CAD build for the part. Positions are in the model's coordinates, mm. A direction names the side the tool comes from. Coordinates: 2 decimals unless noted, no trailing zeros. Order: outer loops, then holes, each group sorted by start corner. A loop starts at its lowest first (then second) coordinate and runs counter-clockwise, first axis right, second up. Notation, with made-up numbers: M 12.25,15 L 35.25,15 A7 ccw 35.25,27 Z; hole C 45.5,25.5 d3. An arc over 180 degrees is marked long. One line per item, written item: value.
Autodesk Inventor part; units mm, degrees
ref_plane "YZ Plane" through (0, 0, 0) normal (1, 0, 0) x (0, 1, 0)
ref_plane "XZ Plane" through (0, 0, 0) normal (0, 1, 0) x (-1, 0, 0)
ref_plane "XY Plane" through (0, 0, 0) normal (0, 0, 1) x (1, 0, 0)
sketch "Sketch1" plane through (0, 0, 0) normal (0, 0, 1) x (1, 0, 0)
  point P0 (0, 0)
sketch "Sketch2" plane through (0, 0, 0) normal (0, 0, 1) x (1, 0, 0)
  line L0 (76.1957, 14.1695) -> (-73.6643, 14.1695) construction
  line L1 (-73.6643, -54.4105) -> (76.1957, -54.4105) construction
  line L2 (34.477, 19.1695) -> (24.477, 19.1695)
  line L3 (24.477, -59.4105) -> (34.477, -59.4105)
  line L4 (34.477, -59.4105) -> (34.477, 19.1695)
  line L5 (24.477, -15.1205) -> (-78.6643, -15.1205)
  line L6 (-78.6643, -15.1205) -> (-78.6643, -25.1205)
  line L7 (-78.6643, -25.1205) -> (24.477, -25.1205)
  line L8 (-73.6643, 14.1695) -> (-73.6643, -54.4105) construction
  line L9 (76.1957, -54.4105) -> (76.1957, 14.1695) construction
  line L10 (76.1957, -20.1205) -> (-73.6643, -20.1205) construction
  line L11 (24.477, 19.1695) -> (24.477, -15.1205)
  line L12 (24.477, -25.1205) -> (24.477, -59.4105)
  line L13 (44.477, -30.2805) -> (44.477, -9.9605) construction
  line L14 (57.177, -30.2805) -> (44.477, -30.2805) construction
  line L15 (57.177, -9.9605) -> (57.177, -30.2805) construction
  line L16 (44.477, -9.9605) -> (57.177, -9.9605) construction
  point P0 (0, 0)
  point P1 (-78.6643, -20.1205)
  dimension "d0" = 5
  dimension "d1" = 5
  dimension "d2" = 5
  dimension "d3" = 10
  dimension "d5" = 10
  dimension "d6" = 10
extrude "Extrusion1" add sketch "Sketch2" along normal blind 5
sketch "Sketch3" plane through (0, 0, 0) normal (0, 0, -1) x (-1, 0, 0)
  line L0 (-76.1957, 14.1695) -> (73.6643, 14.1695)
  line L1 (-76.1957, -54.4105) -> (-76.1957, 14.1695)
  line L2 (73.6643, -54.4105) -> (-76.1957, -54.4105)
  line L3 (73.6643, 14.1695) -> (73.6643, -54.4105)
  line L4 (-34.477, -59.4105) -> (-34.477, 19.1695)
  line L5 (-24.477, 19.1695) -> (-24.477, -15.1205)
  line L6 (-34.477, 19.1695) -> (-24.477, 19.1695)
  line L7 (-24.477, 19.1695) -> (-24.477, 14.1695)
  line L8 (-24.477, 14.1695) -> (-34.477, 14.1695)
  line L9 (-34.477, 14.1695) -> (-34.477, 19.1695)
  line L10 (-24.477, -25.1205) -> (-24.477, -59.4105)
  line L11 (-24.477, -59.4105) -> (-34.477, -59.4105)
  line L12 (-34.477, -59.4105) -> (-34.477, -54.4105)
  line L13 (-34.477, -54.4105) -> (-24.477, -54.4105)
  line L14 (-24.477, -54.4105) -> (-24.477, -59.4105)
  line L15 (73.6643, 22.9533) -> (78.6643, 22.9533)
  line L16 (78.6643, 22.9533) -> (78.6643, -64.1223)
  line L17 (78.6643, -64.1223) -> (73.6643, -64.1223)
  line L18 (73.6643, -64.1223) -> (73.6643, 22.9533)
  point P0 (0, 0)
  point P1 (-24.477, -54.4105)
  point P2 (-34.477, -54.4105)
  point P3 (-34.477, 14.1695)
extrude "Extrusion2" add sketch "Sketch3" along normal blind 12.9375 contours L4 L6 L5 L0 | L2 L10 L11 L4 | L18 L15 L16 L17 L3
sketch "Sketch4" plane through (0, 0, 0) normal (0, 0, 1) x (1, 0, 0)
  line L0 (-78.6643, -64.1223) -> (-78.6643, 22.9533)
  line L1 (-78.6643, 22.9533) -> (-73.6643, 22.9533)
  line L2 (-73.6643, 22.9533) -> (-73.6643, -64.1223)
  line L3 (-73.6643, -64.1223) -> (-78.6643, -64.1223)
  line L4 (-78.6643, -64.1223) -> (-78.6643, 22.9533)
  point P0 (0, 0)
extrude "Extrusion3" add sketch "Sketch4" along normal blind 5
equation "\"d5\" = d3"
properties part number "Holder"
Q1. Slice it at B-B (y = -27). List the corners of the cut face in (x, z), plus the area to 3 significant figures.
Recorded:
outline: M -78.66,-12.94 L -73.66,-12.94 L -73.66,5 L -78.66,5 Z; M 24.48,0 L 34.48,0 L 34.48,5 L 24.48,5 Z
area: 140 mm^2
Q2. Slice it at A-A (z = -3.25). List the corners of the cut face in (x, y), plus the area to 3 significant figures.
Recorded:
outline: M -78.66,-64.12 L -73.66,-64.12 L -73.66,22.95 L -78.66,22.95 Z; M 24.48,-59.41 L 34.48,-59.41 L 34.48,-54.41 L 24.48,-54.41 Z; M 24.48,14.17 L 34.48,14.17 L 34.48,19.17 L 24.48,19.17 Z
area: 535 mm^2
Q3. Which spindle directions (+Z, -Z, +X, -X, +Y, -Y) get a long thin tool onto all of the face, cutting with end or side? Do faces 4 (the face through (30, 19.17, -4)), 5 (the face through (30, 14.17, -6)), 6 (the face through (-25, -25.12, 2)), 7 (the face through (-24, -15.12, 2)). Say none if no direction does.
Recorded:
face 4: +Z, -Z, +X, +Y
face 5: -Z, +X
face 6: +Z, -Z, -Y
face 7: +Z, -Z, +Y
Q4. Slice it at C-C (x = 26.5). List the corners of the cut face in (y, z).
Recorded:
outline: M -59.41,-12.94 L -54.41,-12.94 L -54.41,0 L 14.17,0 L 14.17,-12.94 L 19.17,-12.94 L 19.17,5 L -59.41,5 Z
Q5. Pin check, flat tips, straight feed: pin 1 Ø4 at (x, z) = (-25.5, 2.5) entering from +Y; pin 2 Ø20.5 at (x, y) = (-21.5, -9) entering from -Z; pin 3 Ø2.5 at (x, z) = (-11, 1.5) entering from -Y; pin 4 Ø10 at (x, z) = (-41, -7.5) entering from +Y. Stop position of each tip, or through.
Recorded:
pin 1: stops at y = -15.12
pin 2: stops at z = 0
pin 3: stops at y = -25.12
pin 4: passes through
Q6. Mould opens along Y. For faces 1 (the face through (-18, -24, 5)), 2 (the face through (-4, -20, 0)), 3 (the face through (-76, 22.953, -4)) say: released by +Y, released by -Y, zero draft, split by the parting line, or undercut.
Recorded:
face 1: zero draft
face 2: undercut
face 3: released by +Y
Q7. Drill centre lines: line 1 along X through (y, z) = (-50, 0.5); line 2 along X through (y, z) = (-31, -8); line 3 along Y through (x, z) = (18.5, 4). Where is each one in solid material? Low to high.
Recorded:
line 1: x = -78.66 to -73.66, 24.48 to 34.48
line 2: x = -78.66 to -73.66
line 3: y = -25.12 to -15.12
Q8. Slice it at D-D (z = 2.5). List the corners of the cut face in (x, y).
Recorded:
outline: M -78.66,-64.12 L -73.66,-64.12 L -73.66,-25.12 L 24.48,-25.12 L 24.48,-59.41 L 34.48,-59.41 L 34.48,19.17 L 24.48,19.17 L 24.48,-15.12 L -73.66,-15.12 L -73.66,22.95 L -78.66,22.95 Z
